Source: CAD feature listing. Evaluate the final solid. Frame: model axes, mm. Give positions to 0.01 mm unless a question says otherwise; leave off trailing zeros. Write each loop counter-clockwise with the first axis right and the second up, starting at its lowest first coordinate (ties: lowest second). Pieces come first, ordered by that corner, then holes. Notation, with made-up numbers: M 78,-33.75 L 124,-33.75 A9 ccw 124,-25.75 Z; hole C 27,31 d5. An arc over 180 degrees is marked long. Answer as a JSON object with one key per item and string values. Group by question number.
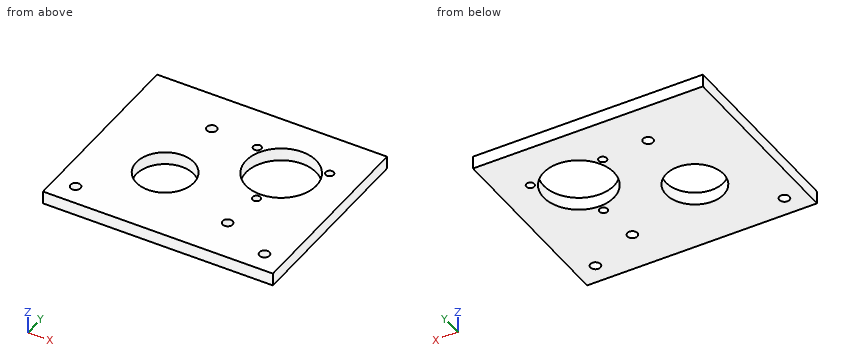
Autodesk Inventor part; units mm, degrees
ref_plane "Work Plane1" through (0, 0, -6.35) normal (0, 0, 1) x (1, 0, 0)
ref_plane "Work Plane2" through (0, 0, -41.875) normal (0, 0, 1) x (1, 0, 0)
ref_plane "Work Plane3" through (0, 0, -35.525) normal (0, 0, 1) x (1, 0, 0)
sketch "Sketch1" plane through (0, 0, 0) normal (0, 0, 1) x (1, 0, 0)
  line L0 (0, 0) -> (114.0582, 0)
  line L1 (114.0582, 0) -> (114.0582, 95.9104)
  line L2 (114.0582, 95.9104) -> (0, 95.9104)
  line L3 (0, 95.9104) -> (0, 0)
  line L4 (59.1, 17.1) -> (59.1, 59.1)
  line L5 (59.1, 59.1) -> (17.1, 59.1)
  line L6 (17.1, 59.1) -> (17.1, 17.1)
  line L7 (17.1, 17.1) -> (59.1, 17.1)
  line L8 (59.1, 17.1) -> (17.1, 59.1) construction
  line L9 (59.1, 59.1) -> (17.1, 17.1) construction
  circle A0 centre (38.1, 38.1) radius 38.1 construction
  circle A1 centre (38.1, 38.1) radius 20.2
  line L10 (45.4323, 38.1) -> (41.7662, 31.75)
  line L11 (41.7662, 31.75) -> (34.4338, 31.75)
  line L12 (34.4338, 31.75) -> (30.7677, 38.1)
  line L13 (30.7677, 38.1) -> (34.4338, 44.45)
  line L14 (34.4338, 44.45) -> (41.7662, 44.45)
  line L15 (41.7662, 44.45) -> (45.4323, 38.1)
  circle A2 centre (38.1, 38.1) radius 21.59 construction
  line L16 (38.1, 38.1) -> (81.0382, 62.8904) construction
  circle A3 centre (81.0382, 62.8904) radius 27.94 construction
  circle A4 centre (81.0382, 62.8904) radius 23.8125 construction
  circle A5 centre (81.0382, 62.8904) radius 17.4625
  circle A6 centre (38.1, 38.1) radius 14.2875
  line L17 (85.0105, 18.6054) -> (38.1, 38.1) construction
  circle A7 centre (81.0382, 62.8904) radius 33.02 construction
  circle A8 centre (38.1, 38.1) radius 25.4 construction
  circle A9 centre (38.1, 38.1) radius 9.525
  line L18 (81.0382, 62.8904) -> (81.0382, 42.1545)
  circle A10 centre (81.0382, 42.1545) radius 2.0828 construction
  circle A11 centre (39.5622, 74.901) radius 10.16
  circle A12 centre (39.5622, 74.901) radius 6.35
  circle A13 centre (81.0382, 42.1545) radius 6.35 construction
  circle A14 centre (38.1, 38.1) radius 26.67 construction
  line L19 (85.0105, 18.6054) -> (87.4474, 24.4692)
  line L20 (85.0105, 18.6054) -> (82.5737, 12.7416)
  line L21 (87.4474, 24.4692) -> (77.6267, 28.5504)
  line L22 (82.5737, 12.7416) -> (72.2567, 17.029)
  circle A15 centre (103.8982, 10.16) radius 10.16
  circle A16 centre (103.8982, 10.16) radius 6.35
  circle A17 centre (10.16, 10.16) radius 10.16
  circle A18 centre (38.1, 38.1) radius 32.258 construction
  circle A19 centre (10.16, 10.16) radius 6.35
  point P0 (20.1395, 56.0605)
  point P1 (56.0605, 20.1395)
  point P2 (81.0382, 44.2373)
  point P3 (81.0382, 45.4279)
  point P4 (98.9961, 73.2584)
  point P5 (63.0804, 73.2584)
  point P6 (81.0382, 48.5045)
  point P7 (79.1467, 21.0422)
  dimension "d10" = 34.925
  dimension "d17" = 4.1656
  dimension "d25" = 12.7
  dimension "d0" = 42
  dimension "d1" = 42
  dimension "d2" = 76.2
  dimension "d3" = 40.4
  dimension "d4" = 12.7
  dimension "d5" = 43.18
  dimension "d6" = 55.88
  dimension "d7" = 49.5808
  dimension "d8" = 47.625
  dimension "d11" = 28.575
  dimension "d13" = 30
  dimension "d14" = 5.08
  dimension "d15" = 50.8
  dimension "d16" = 19.05
  dimension "d18" = 1.1906
  dimension "d21" = 360
  dimension "d23" = 20.32
  dimension "d24" = 12.7
  dimension "d26" = 3.0766
  dimension "d30" = 5.08
  dimension "d33" = 50.8
  dimension "d34" = 6.35
  dimension "d35" = 6.35
  dimension "d36" = 20.32
  dimension "d37" = 64.516
  dimension "d38" = 12.7
ref_plane "Work Plane1" through (0, 0, -6.35) normal (0, 0, 1) x (1, 0, 0)
ref_plane "Work Plane2" through (0, 0, -41.875) normal (0, 0, 1) x (1, 0, 0)
ref_plane "Work Plane3" through (0, 0, -35.525) normal (0, 0, 1) x (1, 0, 0)
ref_plane "Work Plane4" through (0, 0, -92.675) normal (0, 0, 1) x (1, 0, 0)
ref_plane "Work Plane5" through (0, 0, -99.025) normal (0, 0, 1) x (1, 0, 0)
sketch "Sketch2" plane through (0, 0, -6.35) normal (0, 0, 1) x (1, 0, 0)
  line L0 (114.0582, 95.9104) -> (0, 95.9104)
  line L1 (0, 95.9104) -> (0, 0)
  line L2 (0, 0) -> (114.0582, 0)
  line L3 (114.0582, 0) -> (114.0582, 95.9104)
  circle A0 centre (81.0382, 62.8904) radius 17.4625
  circle A1 centre (38.1, 38.1) radius 9.525
  dimension "d14" = 5.08
sketch "Sketch3" plane through (0, 0, -41.875) normal (0, 0, 1) x (1, 0, 0)
  line L0 (114.0582, 95.9104) -> (0, 95.9104)
  line L1 (114.0582, 0) -> (114.0582, 95.9104)
  circle A0 centre (81.0382, 62.8904) radius 17.4625
  line L2 (0, 0) -> (114.0582, 0)
  line L3 (0, 95.9104) -> (0, 0)
  circle A1 centre (38.1, 38.1) radius 14.2875
  dimension "d14" = 5.08
sketch "Sketch4" plane through (0, 0, -35.525) normal (0, 0, 1) x (1, 0, 0)
  line L0 (114.0582, 95.9104) -> (0, 95.9104)
  line L1 (0, 95.9104) -> (0, 0)
  line L2 (0, 0) -> (114.0582, 0)
  line L3 (114.0582, 0) -> (114.0582, 95.9104)
  circle A0 centre (81.0382, 62.8904) radius 17.4625
  circle A1 centre (38.1, 38.1) radius 14.2875
  dimension "d14" = 5.08
sketch "Sketch5" plane through (0, 0, -92.675) normal (0, 0, 1) x (1, 0, 0)
  line L0 (0, 95.9104) -> (0, 0)
  line L1 (114.0582, 95.9104) -> (0, 95.9104)
  line L2 (0, 0) -> (114.0582, 0)
  line L3 (114.0582, 0) -> (114.0582, 95.9104)
  circle A0 centre (81.0382, 62.8904) radius 17.4625
  dimension "d14" = 5.08
sketch "Sketch6" plane through (0, 0, -99.025) normal (0, 0, 1) x (1, 0, 0)
  line L0 (0, 95.9104) -> (0, 0)
  line L1 (0, 0) -> (114.0582, 0)
  line L2 (114.0582, 0) -> (114.0582, 95.9104)
  line L3 (114.0582, 95.9104) -> (0, 95.9104)
  circle A0 centre (81.0382, 62.8904) radius 17.4625
  dimension "d14" = 5.08
extrude "Extrusion1" add sketch "Sketch1" along normal blind 6.35 contours L3 A17 L0 | A17 L7 L4 L5 L6 L3 L2 L1 A15 L0 | A17 L6 L7 | A15 L1 L0 | A15 | A17 L7 L6 | L6 L5 L4 L7 A17 | A1 | A11 | A12 | A16 | A19
hole "Hole1" at (81.0382, 42.1545, 0) at (98.9961, 73.2584, 0) at (63.0804, 73.2584, 0) direction (0, 0, 1) diameter 3.9624 end through all
hole "Hole2" at (79.1467, 21.0422, 0) direction (0, 0, 1) diameter 4.9784 end through all
hole "Hole3" at (39.5622, 74.901, 0) at (103.8982, 10.16, 0) at (10.16, 10.16, 0) direction (0, 0, 1) diameter 4.9784 end through all
equation "\"d30\" = d14"
properties part number "Main Outline"
(1) Section A-A, the plane x = 10.16. Return loops of the section in (y, z), plus the area to 3 significant figures.
(2) Contact query for a flat-ended pin moving along its axis: pin 1 Ø6.5 at (x, y) = (39.56, 74.9) entering from -Z. Output: stop coordinate, or through.
(3) Section B-B, the plane y = 10.16. Return loops of the section in (x, z), plus the area to 3 significant figures.
(4) Section C-C, the plane y = 70. Return loops of the section in (x, z), plus the area to 3 significant figures.
(5) Section D-D, the plane y = 48. Return loops of the section in (x, z).
(6) Ray query, L1, parallel to X at y = 10.16, z = 4.5; L2, parallel to X at y = 9.5, z = 5.75; L3, parallel to X at y = 73, z = 4.75. Return the intervals inside material, ascending. Write a range as [from, to].
Reported:
{
 "1": {"outline": "M 0,0 L 7.67,0 L 7.67,6.35 L 0,6.35 Z; M 12.65,0 L 95.91,0 L 95.91,6.35 L 12.65,6.35 Z", "area": "577 mm2"},
 "2": {"pin 1": "stops at z = 0"},
 "3": {"outline": "M 0,0 L 7.67,0 L 7.67,6.35 L 0,6.35 Z; M 12.65,0 L 101.41,0 L 101.41,6.35 L 12.65,6.35 Z; M 106.39,0 L 114.06,0 L 114.06,6.35 L 106.39,6.35 Z", "area": "661 mm2"},
 "4": {"outline": "M 0,0 L 65.09,0 L 65.09,6.35 L 0,6.35 Z; M 96.99,0 L 114.06,0 L 114.06,6.35 L 96.99,6.35 Z", "area": "522 mm2"},
 "5": {"outline": "M 0,0 L 27.8,0 L 27.8,6.35 L 0,6.35 Z; M 48.4,0 L 71.92,0 L 71.92,6.35 L 48.4,6.35 Z; M 90.16,0 L 114.06,0 L 114.06,6.35 L 90.16,6.35 Z"},
 "6": {"L1": "x = [0, 7.67], [12.65, 101.41], [106.39, 114.06]", "L2": "x = [0, 7.76], [12.56, 101.5], [106.3, 114.06]", "L3": "x = [0, 37.96], [41.17, 61.12], [65.04, 66.8], [95.28, 97.03], [100.96, 114.06]"}
}
